Geometry check sheet. Reference: drawing and pictorial views, mm from the part's lowest x, y, z. A direction names the side the tool comes from. Give positions to 0.01 mm unless a question says otherwise; leave off trailing zeros. Order: outer loops, then holes, each group sorted by start corner. A loop starts at its lowest first (then second) coordinate and runs counter-clockwise, first axis right, second up.
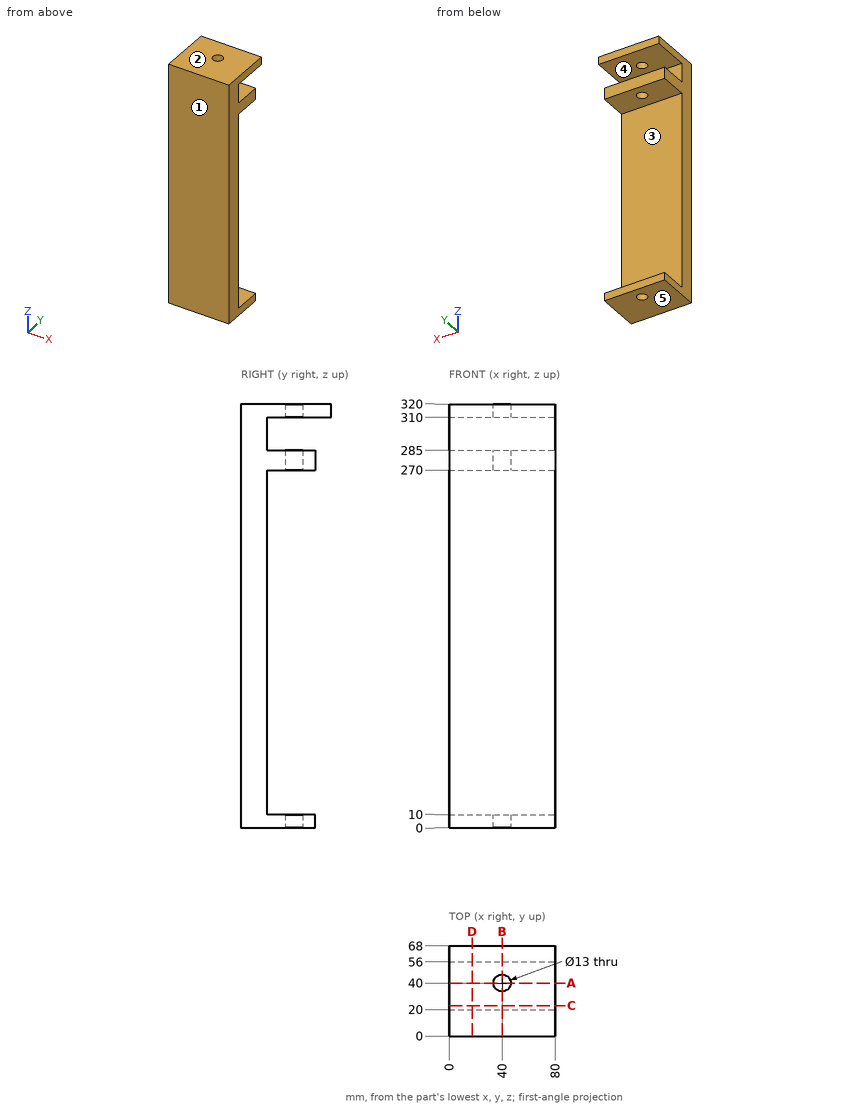
1) Draft check along Z on the marked faces 1, 2 and 3. Enter one of: +Z half, -Z half, draft (parallel to the pull), parting line (faces both ways), or undercut.
Recorded:
face 1: draft
face 2: +Z half
face 3: undercut
2) Set-up check for the marked faces 4 and 5: record each of +Z, -Z, +X, -X, +Y, -Y from which the full face is reachable in a straight line by a thin tool's end or side.
Recorded:
face 4: +X, -X, +Y
face 5: -Z, +X, -X, +Y, -Y
3) Section check A-A, the plane y = 40. Record the cut outline in (x, z).
Recorded:
outline: (0, 0) - (33.5, 0) - (33.5, 10) - (0, 10) - close; (0, 270) - (33.5, 270) - (33.5, 285) - (0, 285) - close; (0, 310) - (33.5, 310) - (33.5, 320) - (0, 320) - close; (46.5, 0) - (80, 0) - (80, 10) - (46.5, 10) - close; (46.5, 270) - (80, 270) - (80, 285) - (46.5, 285) - close; (46.5, 310) - (80, 310) - (80, 320) - (46.5, 320) - close
4) Section check C-C, the plane y = 23. Record the cut outline in (x, z), then the cut area to 3 significant figures.
Recorded:
outline: (0, 0) - (80, 0) - (80, 10) - (0, 10) - close; (0, 270) - (80, 270) - (80, 285) - (0, 285) - close; (0, 310) - (80, 310) - (80, 320) - (0, 320) - close
area: 2,800 mm2
5) Depth check by flat-ended pin: pin 1 Ø16.5 at (x, z) = (23.5, 279.5) entering from +Y; pin 2 Ø1 at (x, z) = (16, 114.5) entering from +Y. Enter the tip coordinate at first touch or a pass-through.
Recorded:
pin 1: stops at y = 56
pin 2: stops at y = 20
6) Material ranges on L1, parallel to Z at x = 16, y = 39; L2, parallel to Y at x = 40, z = 313; L3, parallel to Y at x = 40, z = 275.25, recorded low to high.
Recorded:
L1: z = 0 to 10, 270 to 285, 310 to 320
L2: y = 0 to 33.5, 46.5 to 68
L3: y = 0 to 33.5, 46.5 to 56
7) Section check B-B, the plane x = 40. Record the cut outline in (y, z), then the cut area to 4 significant figures.
Recorded:
outline: (0, 0) - (33.5, 0) - (33.5, 10) - (20, 10) - (20, 270) - (33.5, 270) - (33.5, 285) - (20, 285) - (20, 310) - (33.5, 310) - (33.5, 320) - (0, 320) - close; (46.5, 0) - (56, 0) - (56, 10) - (46.5, 10) - close; (46.5, 270) - (56, 270) - (56, 285) - (46.5, 285) - close; (46.5, 310) - (68, 310) - (68, 320) - (46.5, 320) - close
area: 7,325 mm2
8) Section check D-D, the plane x = 17.5. Record the cut outline in (y, z).
Recorded:
outline: (0, 0) - (56, 0) - (56, 10) - (20, 10) - (20, 270) - (56, 270) - (56, 285) - (20, 285) - (20, 310) - (68, 310) - (68, 320) - (0, 320) - close
